Study the drawing (mm; zero at the part's minimum x, y, z) and answer. A direction names the side the tool comes from. Coordinates: 2 decimals unless noted, no trailing zeros. Loops run counter-clockwise (first coordinate to the right, second up) from the corner with the lowest first, then second, coordinate; pieces in that order, holes last. Notation, with made-up numbers: (-27, -15) - (10, -15) arc R18 ccw to (10, 10) - close; hole circle Ø11 at (6, 42.25). An arc over 180 degrees is marked (long way). One line per item, written item: value. Start each with the question number.
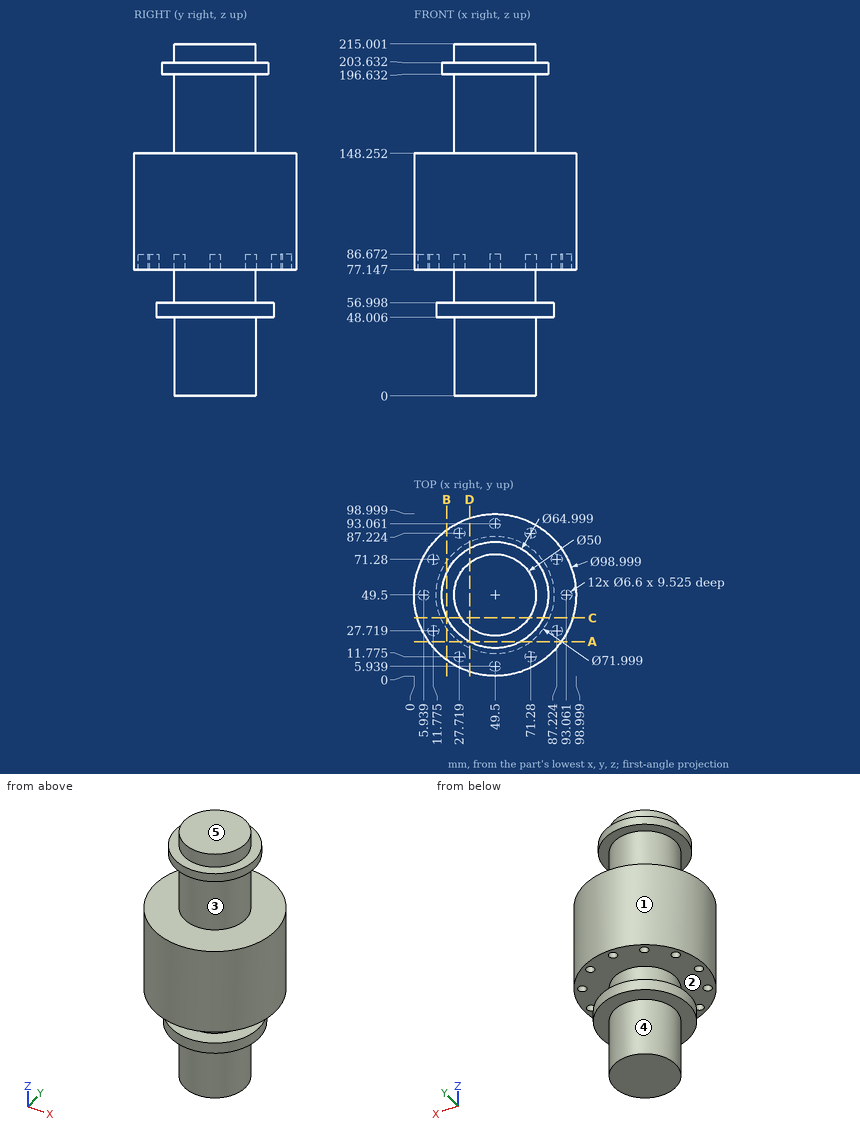
1) Determine the mould class of the marked faces 3, 4 and 5 for opening direction Z: released by +Z, released by -Z, zero draft, split by the parting line, or undercut.
2) For the marked faces 1 and 2, determine the directions among +Z, -Z, +X, -X, +Y, -Y from which every point of the face is accessible in a straight line to the end or side of a thin tool.
3) Straight lines are drawn through the part: L1, parallel to Z at x = 56, y = 22.5; L2, parallel to Z at x = 19, y = 68; L3, parallel to Z at x = 90, y = 35. For each, find the intervals that lie inside material, in ascending order.
4) Section D-D, the plane x = 34 is taken. Determine the outline of the cut face in (y, z) (1 decimal), and give its area (3 significant figures).
5) Flat-ended cylindrical pins translate along their axes: P1, Ø6, axis at x = 93.06, y = 49.5, coming from the +Z side; P2, Ø4, axis at x = 5.94, y = 49.5, coming from the -Z side; P3, Ø10, axis at y = 61, z = 57.5, coming from the -X side; P4, Ø8, axis at y = 18, z = 192, coming from the +X side. Find the tip coordinate at first contact, or state that the pin passes through.
6) Section C-C, the plane y = 35.5 is taken. Determine the outline of the cut face in (x, z) (1 decimal).
7) Section B-B, the plane x = 20 is taken. Determine the outline of the cut face in (y, z).
8) Section A-A, the plane y = 21 is taken. Determine the outline of the cut face in (x, z) (1 decimal), and give its area (3 significant figures).
Answer below:
1. face 3: undercut
1. face 4: zero draft
1. face 5: released by +Z
2. face 1: +Z, -Z
2. face 2: none
3. L1: 48.01 to 57, 77.15 to 148.25, 196.63 to 203.63
3. L2: 48.01 to 57, 77.15 to 148.25
3. L3: 77.15 to 148.25
4. outline: (2.5, 77.1) - (29.9, 77.1) - (29.9, 57) - (17, 57) - (17, 48) - (29.9, 48) - (29.9, 0) - (69.1, 0) - (69.1, 48) - (82, 48) - (82, 57) - (69.1, 57) - (69.1, 77.1) - (96.5, 77.1) - (96.5, 148.3) - (69.1, 148.3) - (69.1, 196.6) - (78.1, 196.6) - (78.1, 203.6) - (69.1, 203.6) - (69.1, 215) - (29.9, 215) - (29.9, 203.6) - (20.9, 203.6) - (20.9, 196.6) - (29.9, 196.6) - (29.9, 148.3) - (2.5, 148.3) - close
4. area: 12,700 mm2
5. P1: z = 148.25
5. P2: z = 86.67
5. P3: x = 14.1
5. P4: through
6. outline: (2, 77.1) - (28.8, 77.1) - (28.8, 57) - (16.3, 57) - (16.3, 48) - (28.8, 48) - (28.8, 0) - (70.2, 0) - (70.2, 48) - (82.7, 48) - (82.7, 57) - (70.2, 57) - (70.2, 77.1) - (97, 77.1) - (97, 148.3) - (70.2, 148.3) - (70.2, 196.6) - (78.8, 196.6) - (78.8, 203.6) - (70.2, 203.6) - (70.2, 215) - (28.8, 215) - (28.8, 203.6) - (20.2, 203.6) - (20.2, 196.6) - (28.8, 196.6) - (28.8, 148.3) - (2, 148.3) - close
7. outline: (9.75, 77.15) - (89.25, 77.15) - (89.25, 148.25) - (9.75, 148.25) - close; (28.87, 48.01) - (70.13, 48.01) - (70.13, 57) - (28.87, 57) - close; (35.86, 196.63) - (63.14, 196.63) - (63.14, 203.63) - (35.86, 203.63) - close
8. outline: (9, 77.1) - (90, 77.1) - (90, 148.3) - (9, 148.3) - close; (27.5, 48) - (71.5, 48) - (71.5, 57) - (27.5, 57) - close; (33.9, 196.6) - (65.1, 196.6) - (65.1, 203.6) - (33.9, 203.6) - close
8. area: 6,370 mm2
